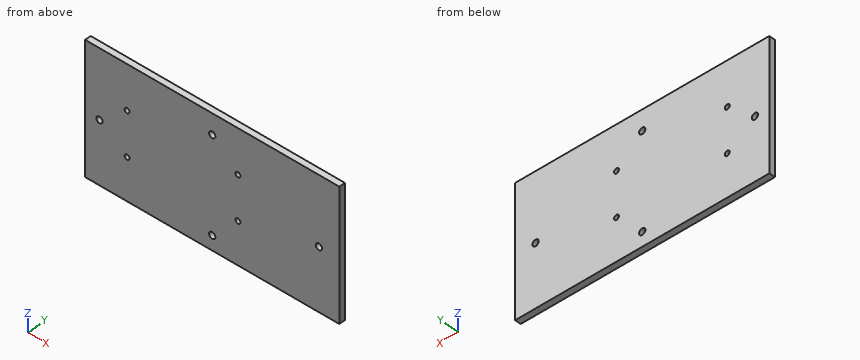
from build123d import *

# Parameters (mm, degrees)
SKETCH1_W           = 133.175
SKETCH1_H           = 68.175
SKETCH1_R           = 1.65
BOSS_EXTRUDE1_DEPTH = 3.175
SKETCH2_R           = 1.3
CUT_EXTRUDE1_DEPTH  = 3.175


with BuildPart() as part:
    # Sketch1 → Boss-Extrude1 (new body)
    with BuildSketch(Plane(origin=(0, 0, 0), x_dir=(1, 0, 0), z_dir=(0, 1, 0))):
        Rectangle(SKETCH1_W, SKETCH1_H)
        with Locations(Location((0, 26.5875, 0), (0, 0, 270))):
            Circle(SKETCH1_R, mode=Mode.SUBTRACT)
        with Locations(Location((-59.0875, 1.5875, 0), (0, 0, 270))):
            Circle(SKETCH1_R, mode=Mode.SUBTRACT)
        with Locations(Location((55.9125, 1.5875, 0), (0, 0, 270))):
            Circle(SKETCH1_R, mode=Mode.SUBTRACT)
        with Locations(Location((0, -23.4125, 0), (0, 0, 270))):
            Circle(SKETCH1_R, mode=Mode.SUBTRACT)
    extrude(amount=BOSS_EXTRUDE1_DEPTH)

    # Sketch2 → Cut-Extrude1 (cut)
    with BuildSketch(Plane.XZ):
        with Locations(Location((-44.5875, 10.9625, 0), (0, 0, 270))):
            Circle(SKETCH2_R)
        with Locations(Location((-44.5875, -12.0875, 0), (0, 0, 270))):
            Circle(SKETCH2_R)
        with Locations(Location((13.4625, -12.0875, 0), (0, 0, 270))):
            Circle(SKETCH2_R)
        with Locations(Location((13.4625, 10.9625, 0), (0, 0, 270))):
            Circle(SKETCH2_R)
    extrude(amount=-CUT_EXTRUDE1_DEPTH, mode=Mode.SUBTRACT)


solid = part.part
Geometry check sheet. Reference: the model listing, model coordinates, mm. Coordinates: 2 decimals unless noted, no trailing zeros. Write each loop counter-clockwise with the first axis right and the second up, starting at its lowest first coordinate (ties: lowest second). Pieces come first, ordered by that corner, then holes. Notation, with made-up numbers: (-31.5, -14) -> (-2.5, -14) arc R22 cw to (-2.5, 3) -> close; hole circle Ø8 at (63.5, -37.75). An arc over 180 degrees is marked (long way). One line per question, with ' | ' between items.
1. Cross-section at A-A on x = 0. Record the cut outline in (y, z) (1 decimal), and give its area (3 significant figures).
Answers:
outline: (0, -34.1) -> (3.2, -34.1) -> (3.2, -28.2) -> (0, -28.2) -> close; (0, -24.9) -> (3.2, -24.9) -> (3.2, 21.8) -> (0, 21.8) -> close; (0, 25.1) -> (3.2, 25.1) -> (3.2, 34.1) -> (0, 34.1) -> close | area: 196 mm²
2. Cross-section at B-B on z = -12. Record the cut outline in (x, y) (1 decimal).
Answers:
outline: (-66.6, 0) -> (-45.9, 0) -> (-45.9, 3.2) -> (-66.6, 3.2) -> close; (-43.3, 0) -> (12.2, 0) -> (12.2, 3.2) -> (-43.3, 3.2) -> close; (14.8, 0) -> (66.6, 0) -> (66.6, 3.2) -> (14.8, 3.2) -> close
3. Thickness scan on probe 1 along X at (y, z) = (0.45, -3); probe 2 along Z at (x, y) = (-45.5, 0.45); probe 3 along X at (y, z) = (2.2, -11). Record the ranges inside material, lowest first. Write a range as from..to.
Answers:
probe 1: x = -66.59..-59.94, -58.23..55.06, 56.77..66.59 | probe 2: z = -34.09..-13.01, -11.16..10.04, 11.89..34.09 | probe 3: x = -66.59..-45.3, -43.88..12.75, 14.17..66.59
4. Depth check by flat-ended pin: pin 1 Ø2 at (x, z) = (-44.59, 10.96) entering from -Y (1 decimal). Enter the tip coordinate at first touch or a pass-through.
Answers:
pin 1: passes through
